Autodesk Inventor part; units mm, degrees
ref_plane "YZ Plane" through (0, 0, 0) normal (1, 0, 0) x (0, 1, 0)
ref_plane "XZ Plane" through (0, 0, 0) normal (0, 1, 0) x (-1, 0, 0)
ref_plane "XY Plane" through (0, 0, 0) normal (0, 0, 1) x (1, 0, 0)
sketch "Sketch1" plane through (0, 0, 0) normal (0, 1, 0) x (-1, 0, 0)
  line L0 (0, 17.5) -> (0, 11.5)
  line L1 (0, 11.5) -> (17.5, 11.5)
  line L2 (17.5, 11.5) -> (17.5, 0)
  line L3 (17.5, 0) -> (17.5, -11.5)
  line L4 (17.5, -11.5) -> (0, -11.5)
  line L5 (0, -11.5) -> (0, -17.5)
  line L6 (0, -17.5) -> (20.5, -17.5)
  line L7 (20.5, -17.5) -> (20.5, 17.5)
  line L8 (20.5, 17.5) -> (0, 17.5)
  line L9 (0, 0) -> (0, 11.5) construction
  line L10 (0, 0) -> (0, -11.5) construction
  line L11 (8, 17.5) -> (8, 23.5)
  line L12 (8, 23.5) -> (2, 23.5)
  line L13 (2, 23.5) -> (2, 17.5)
  line L14 (2, -17.5) -> (2, -23.5)
  line L15 (2, -23.5) -> (8, -23.5)
  line L16 (8, -23.5) -> (8, -17.5)
  circle A0 centre (5, 20.5) radius 1.1
  circle A1 centre (5, -20.5) radius 1.1
  line L17 (5, 20.5) -> (5, 23.5) construction
  line L18 (5, -20.5) -> (5, -23.5) construction
  line L19 (5, -20.5) -> (5, 20.5) construction
  line L20 (17.5, 11.5) -> (17.5, 13.5)
  line L21 (17.5, 13.5) -> (12.5, 13.5)
  line L22 (12.5, 13.5) -> (12.5, 11.5)
  line L23 (17.5, -11.5) -> (17.5, -13.5)
  line L24 (17.5, -13.5) -> (12.5, -13.5)
  line L25 (12.5, -13.5) -> (12.5, -11.5)
  dimension "d0" = 23
  dimension "d1" = 17.5
  dimension "d2" = 3
  dimension "d4" = 6
  dimension "d16" = 2.2
  dimension "d17" = 2.2
  dimension "d18" = 3
  dimension "d19" = 3
  dimension "d24" = 41
  dimension "d26" = 5
  dimension "d27" = 5
  dimension "d28" = 2
extrude "Extrusion1" add sketch "Sketch1" along normal blind 10 contours L8 L7 L6 L5 L4 L25 L24 L23 L3 L2 L20 L21 L22 L1 L0
sketch "Sketch2" plane through (0, 0, 17.5) normal (1, 0, 0) x (0, 0, -1)
  line L0 (6, 0) -> (6, 10)
  line L1 (0, 10) -> (6, 10)
  line L2 (0, 0) -> (0, 10)
  line L3 (35, 0) -> (35, 10)
  line L4 (29, 10) -> (35, 10)
  line L5 (29, 0) -> (29, 10)
  circle A0 centre (3.6, 6.2) radius 1.25
  circle A1 centre (31.4, 6.2) radius 1.25
  line L6 (3.6, 6.2) -> (3.6, 0) construction
  line L7 (31.4, 6.2) -> (31.4, 0) construction
  line L8 (6, 0) -> (3.6, 0) construction
  line L9 (29, 0) -> (31.4, 0) construction
  line L10 (3.6, 6.2) -> (6, 6.2) construction
  line L11 (31.4, 6.2) -> (29, 6.2) construction
  point P0 (17.5, 0)
  dimension "d7" = 2.5
  dimension "d31" = 27.8
  dimension "d33" = 6.2
extrude "Extrusion2" cut sketch "Sketch2" against normal blind 10
sketch "Sketch3" plane through (0, 10, 0) normal (0, 1, 0) x (1, 0, 0)
  line L0 (0, -11.5) -> (-12.5, -11.5)
  line L1 (-17.5, -13.5) -> (-17.5, 13.5)
  line L2 (-12.5, 11.5) -> (0, 11.5)
  line L3 (0, 17.5) -> (-20.5, 17.5)
  line L4 (-20.5, 17.5) -> (-20.5, -17.5)
  line L5 (-20.5, -17.5) -> (0, -17.5)
  line L6 (-3, -11.7) -> (-5, -11.7)
  line L7 (-5, -11.7) -> (-5, -16.1)
  line L8 (-5, -16.1) -> (-3, -16.1)
  line L9 (-3, -16.1) -> (-3, -11.7)
  line L10 (-3, -11.7) -> (-5, -16.1) construction
  line L11 (-5, -11.7) -> (-3, -16.1) construction
  line L12 (-3, 16.1) -> (-5, 16.1)
  line L13 (-5, 16.1) -> (-5, 11.7)
  line L14 (-5, 11.7) -> (-3, 11.7)
  line L15 (-3, 11.7) -> (-3, 16.1)
  line L16 (-3, 16.1) -> (-5, 11.7) construction
  line L17 (-5, 16.1) -> (-3, 11.7) construction
  line L18 (-12.5, -11.5) -> (-12.5, -13.5)
  line L19 (-12.5, -13.5) -> (-17.5, -13.5)
  line L20 (-17.5, 13.5) -> (-12.5, 13.5)
  line L21 (-12.5, 13.5) -> (-12.5, 11.5)
  line L22 (0, -12.65) -> (0, -15.15)
  line L23 (0, 15.15) -> (0, 12.65)
  line L24 (0, 13.9) -> (-3, 13.9) construction
  line L25 (-3, -13.9) -> (0, -13.9) construction
  point P0 (0, 0)
  dimension "d11" = 4.4
  dimension "d13" = 2
  dimension "d34" = 3
extrude "Extrusion3" cut sketch "Sketch3" against normal blind 7
extrude "Extrusion4" add sketch "Sketch1" along normal blind 2 contours L13 L12 L11 L8 | L16 L15 L14 L6
fillet "Fillet1" radius 3 8 edges at (-2, 1, 17.5) (-2, 1, -17.5) (-8, 1, 17.5) (-8, 1, -17.5) (-2, 1, 23.5) (-8, 1, 23.5) (-8, 1, -23.5) (-2, 1, -23.5)
fillet "Fillet2" radius 1 6 edges at (-17.5, 5, 13.5) (-12.5, 5, 13.5) (-12.5, 5, 11.5) (-17.5, 5, -13.5) (-12.5, 5, -13.5) (-12.5, 5, -11.5)
properties part number "Servo Holder_3DPrint"
Geometry check sheet. Reference: the model listing, model coordinates, mm. A direction names the side the tool comes from. Coordinates: 2 decimals unless noted, no trailing zeros. Order: outer loops, then holes, each group sorted by start corner. A loop starts at its lowest first (then second) coordinate and runs counter-clockwise, first axis right, second up. Notation, with made-up numbers: (-15.5, 22.5) - (15.5, 22.5) arc R25 ccw to (15.5, 58.5) - close; hole circle Ø5 at (6, 5.25). An arc over 180 degrees is marked (long way). Answer in a Markdown table with one row per item. Add a question column.
1) Material ranges on line 1 along Z through (x, y) = (-5, 1.2); line 2 along Z through (x, y) = (-4.25, 4.25); line 3 along X through (y, z) = (9, 12.5), recorded low to high. Write a range as [from, to].
2) Cross-section at C-C, the plane x = -5.5. Record the cut outline in (y, z), then the cut area to 3 significant figures.
3) Set-up check for faces 4 (the flat face through (-4, 7, -11.7)), 5 (the flat face through (-10, 6, -14)), 6 (the flat face through (-18, 10, 3)), 7 (the flat face through (0, 5, 15)), 8 (the cylindrical face through (-17.215, 5.07, 13.199)): record each of +Z, -Z, +X, -X, +Y, -Y from which the full face is reachable in a straight line by a thin tool's end or side.
4) Cross-section at D-D, the plane z = -4.5. Record the cut outline in (x, y), then the cut area to 3 significant figures.
5) Cross-section at A-A, the plane x = -15.75. Record the cut outline in (y, z).
6) Gauge pin test, flat ends, axial feed: P1, Ø5, axis at x = -11.5, y = 4, coming from the -Z side; P2, Ø1.6, axis at x = -4.5, y = 7, coming from the -Z side; P3, Ø1, axis at x = -4, z = -13, coming from the +Y side. Record the tip position at first contact, or that the pin passes through.
7) Release check for a two-part mould opening along X. For faces 1 (the flat face through (0, 4.9, -14.5)), 2 (the flat face through (-5, 2, -19)), 3 (the flat face through (-15, 5, -13.5)) record: +X half, -X half, draft (parallel to the pull), parting line (faces both ways), or undercut.
8) Cross-section at B-B, the plane y = 9.5. State how many separate pieces and enclosed holes the cut face has, then the cut area to 3 significant figures.
Check result:
| question | item | result |
|---|---|---|
| 1 | line 1 | z = [-23.5, -21.6], [-19.4, -11.5], [11.5, 19.4], [21.6, 23.5] |
| 1 | line 2 | z = [-17.5, -16.1], [-11.7, -11.5], [11.5, 11.7], [16.1, 17.5] |
| 1 | line 3 | x = [-20.5, -17.5], [-12.5, -5], [-3, 0] |
| 2 | outline | (0, -23.46) - (2, -23.46) - (2, -21.48) - (0, -21.48) - close; (0, -19.52) - (2, -19.52) - (2, -17.5) - (10, -17.5) - (10, -11.5) - (0, -11.5) - close; (0, 11.5) - (10, 11.5) - (10, 17.5) - (2, 17.5) - (2, 19.52) - (0, 19.52) - close; (0, 21.48) - (2, 21.48) - (2, 23.46) - (0, 23.46) - close; hole circle Ø2.5 at (6.2, -13.9); hole circle Ø2.5 at (6.2, 13.9) |
| 2 | area | 126 mm² |
| 3 | face 4 | +Y |
| 3 | face 5 | +X |
| 3 | face 6 | +Z, -Z, +X, -X, +Y |
| 3 | face 7 | +Z, -Z, +X, +Y, -Y |
| 3 | face 8 | +Y, -Y |
| 4 | outline | (-20.5, 0) - (-17.5, 0) - (-17.5, 10) - (-20.5, 10) - close |
| 4 | area | 30.0 mm² |
| 5 | outline | (0, -17.5) - (10, -17.5) - (10, -13.5) - (0, -13.5) - close; (0, 13.5) - (10, 13.5) - (10, 17.5) - (0, 17.5) - close |
| 6 | P1 | stops at z = -17.67 |
| 6 | P2 | stops at z = -17.5 |
| 6 | P3 | stops at y = 3 |
| 7 | face 1 | +X half |
| 7 | face 2 | draft |
| 7 | face 3 | undercut |
| 8 | separate pieces | 1 |
| 8 | enclosed holes | 2 |
| 8 | area | 278 mm² |
